Geometry check sheet. Reference: the model listing, model coordinates, mm. A direction names the side the tool comes from. Round coordinates to 2 decimals unless told otherwise and drop trailing zeros. Write each loop counter-clockwise with the first axis right and the second up, starting at its lowest first coordinate (ties: lowest second). Pieces come first, ordered by that corner, then holes.
Item 1: Depth check by flat-ended pin: P1, Ø2, axis at y = -4.5, z = 3.5, coming from the -X side; P2, Ø1.3, axis at y = -3.5, z = 2.5, coming from the +X side; P3, Ø2, axis at x = -114, z = 1.5, coming from the -Y side. Enter the tip coordinate at first touch or a pass-through.
Item 2: Cross-section at C-C (x = -65.5). Enter the section's corners in (y, z), then the cut area to 3 significant figures.
Item 3: Scan lines: probe 1 along Y at (x, z) = (-106, 2.55); probe 2 along X at (y, z) = (48.5, 1.7); probe 3 along Y at (x, z) = (-101, 4.25). Record each from-to range of solid material in increasing order.
Item 4: Cross-section at A-A (y = 48). Enter the section's corners in (x, z), then the cut area to 3 significant figures.
Item 5: Draft check along X on faces 5 (the face through (-96.932, -4, 2)), 6 (the face through (-69, -6.115, 2)), 7 (the face through (-61.932, 28, 2)). Enter one of: pulls with the +X half, pulls with the -X half, needs draft (parallel to the pull), parting line crosses it, or undercut.
Item 6: Access from +Z, -Z, +X, -X, +Y, -Y to the whole of each face (thin tool, end or side, straight path). Record for faces 1 (the face through (-64, -1.615, 2)), 2 (the face through (-101.932, -4, 2)), 3 (the face through (-79, -6.115, 2)), 4 (the face through (-115, -1.615, 2)).
Item 7: Cross-section at B-B (z = 2). Enter the section's corners in (x, y).
from build123d import *

# Parameters (mm, degrees)
SKETCH1_R           = 2.5
SKETCH1_W           = 5
SKETCH1_H           = 4.5
BOSS_EXTRUDE1_DEPTH = 4.5


with BuildPart() as part:
    # Sketch1 → Boss-Extrude1 (new body)
    # profile 1 of 5: a face of its own
    with BuildSketch(Plane.XY):
        Polygon((-111.932160423, -1.614828107), (-111.932160423, -6.114828107), (-106.932160423, -6.114828107), (-106.932160423, -1.614828107), (-101.932160423, -1.614828107), (-96.932160423, -1.614828107), (-91.932160423, -1.614828107), (-86.932160423, -1.614828107), (-81.932160423, -1.614828107), (-76.932160423, -1.614828107), (-71.932160423, -1.614828107), (-66.932160423, -1.614828107), (-61.932160423, -1.614828107), (-61.932160423, 58.885171893), (-117.932160423, 58.885171893), (-117.932160423, -1.614828107), align=None)
        with Locations((-102.932160423, 13.885171893)):
            Circle(SKETCH1_R, mode=Mode.SUBTRACT)
        with Locations((-102.932160423, 48.885171893)):
            Circle(SKETCH1_R, mode=Mode.SUBTRACT)
    # profile 2 of 5: a face of its own
    with BuildSketch(Plane.XY):
        with Locations((-99.432160423, -3.864828107)):
            Rectangle(SKETCH1_W, SKETCH1_H)
    # profile 3 of 5: a face of its own
    with BuildSketch(Plane.XY):
        with Locations((-69.432160423, -3.864828107)):
            Rectangle(SKETCH1_W, SKETCH1_H)
    # profile 4 of 5: a face of its own
    with BuildSketch(Plane.XY):
        with Locations((-79.432160423, -3.864828107)):
            Rectangle(SKETCH1_W, SKETCH1_H)
    # profile 5 of 5: a face of its own
    with BuildSketch(Plane.XY):
        with Locations((-89.432160423, -3.864828107)):
            Rectangle(SKETCH1_W, SKETCH1_H)
    extrude(amount=BOSS_EXTRUDE1_DEPTH)


solid = part.part
Resolved:
1. P1: stops at x = -111.93
1. P2: stops at x = -66.93
1. P3: stops at y = -1.61
2. outline: (-1.61, 0) - (58.89, 0) - (58.89, 4.5) - (-1.61, 4.5) - close
2. area: 272 mm2
3. probe 1: y = -1.61 to 58.89
3. probe 2: x = -117.93 to -105.4, -100.46 to -61.93
3. probe 3: y = -6.11 to 12.3, 15.47 to 47.3, 50.47 to 58.89
4. outline: (-117.93, 0) - (-105.27, 0) - (-105.27, 4.5) - (-117.93, 4.5) - close; (-100.59, 0) - (-61.93, 0) - (-61.93, 4.5) - (-100.59, 4.5) - close
4. area: 231 mm2
5. face 5: undercut
5. face 6: needs draft
5. face 7: pulls with the +X half
6. face 1: +Z, -Z, +X, -Y
6. face 2: +Z, -Z, -Y
6. face 3: +Z, -Z, +X, -X, -Y
6. face 4: +Z, -Z, -X, -Y
7. outline: (-117.93, -1.61) - (-111.93, -1.61) - (-111.93, -6.11) - (-106.93, -6.11) - (-106.93, -1.61) - (-101.93, -1.61) - (-101.93, -6.11) - (-96.93, -6.11) - (-96.93, -1.61) - (-91.93, -1.61) - (-91.93, -6.11) - (-86.93, -6.11) - (-86.93, -1.61) - (-81.93, -1.61) - (-81.93, -6.11) - (-76.93, -6.11) - (-76.93, -1.61) - (-71.93, -1.61) - (-71.93, -6.11) - (-66.93, -6.11) - (-66.93, -1.61) - (-61.93, -1.61) - (-61.93, 58.89) - (-117.93, 58.89) - close; hole circle Ø5 at (-102.93, 13.89); hole circle Ø5 at (-102.93, 48.89)
